from build123d import *

# Parameters (mm, degrees)
EXTRUDE_1_DEPTH = 75
FILLET_1_R      = 2


with BuildPart() as part:
    # ｽｹｯﾁ1 → ﾎﾞｽ - 押し出し1 (new body)
    with BuildSketch(Plane(origin=(0, 0, 0), x_dir=(0, 0, -1), z_dir=(1, 0, 0))):
        Polygon((0, 0), (0, -14), (10, -14), (10, -19), (25, -5), (25, 0), align=None)
    extrude(amount=EXTRUDE_1_DEPTH)

    # ﾌｨﾚｯﾄ1
    fillet_1_edges = [part.edges().sort_by_distance(p)[0] for p in [
        (37.5, 0, -25),
        (37.5, -5, -25),
        (37.5, -14, 0),
        (37.5, 0, 0),
    ]]
    fillet(fillet_1_edges, radius=FILLET_1_R)


solid = part.part
The model under review builds one solid part; all positions refer to its coordinate system, in mm. A direction names the side the tool comes from. Round coordinates to 2 decimals unless told otherwise and drop trailing zeros. Loops run counter-clockwise (first coordinate to the right, second up) from the corner with the lowest first, then second, coordinate; pieces in that order, holes last. Notation, with made-up numbers: (87, 56.5) -> (129, 56.5) arc R19 cw to (129, 69.5) -> close; hole circle Ø5 at (52.5, -30). An arc over 180 degrees is marked (long way). Write item = value, one per line. Start each with the question number.
Item 1: Take a section at B-B on z = -9. Give the boundary of the cut face in (x, y).
Item 2: Take a section at C-C on y = -9. Give the boundary of the cut face in (x, z).
Item 3: For faces 1 (the flat face through (37, -16, -10)), 2 (the flat face through (36.98, -12.39, -17.08)), list the 3-axis set-ups (+Z, -Z, +X, -X, +Y, -Y) from which the entire face can be reached by the end or side of a thin tool; tool diameter is ignored.
Item 4: To check wall thickness, follow L1, parallel to Y at x = 67.5, z = -9.25; L2, parallel to Z at x = 42.5, y = -4.25; L3, parallel to Y at x = 8, z = -14. State the ranges of each line that lie inside material, in increasing order.
Item 5: Take a section at A-A on x = 20. Give the boundary of the cut face in (y, z), plus the area to 3 significant figures.
Item 6: Insertion check: pin 1 (2.5 mm diameter, centred on x = 31.5, z = -4.5, fed in from -Y); pin 2 (2.5 mm diameter, centred on x = 25, y = -16, fed in from +Z); pin 3 (3 mm diameter, centred on y = -17, z = -6, fed in from -X); pin 4 (6 mm diameter, centred on x = 12.5, y = -7.5, fed in from -Z). Each pin has a flat end and moves straight along its axis. Give the tip position at first contact, or say it passes through.
Result:
q1.outline = (0, -14) -> (75, -14) -> (75, 0) -> (0, 0) -> close
q2.outline = (0, -20.71) -> (75, -20.71) -> (75, 0) -> (0, 0) -> close
q3.face_1 = +Z, +X, -X, -Y
q3.face_2 = -Z, +X, -X, -Y
q4.L1 = -14 to 0
q4.L2 = -25 to 0
q4.L3 = -15.27 to 0
q5.outline = (-19, -10) -> (-5.59, -24.36) arc R2 ccw to (-4.13, -25) -> (-2, -25) arc R2 ccw to (0, -23) -> (0, -2) arc R2 ccw to (-2, 0) -> (-12, 0) arc R2 ccw to (-14, -2) -> (-14, -10) -> close
q5.area = 317 mm²
q6.pin_1 = -14
q6.pin_2 = -10
q6.pin_3 = through
q6.pin_4 = -24.97
